Could you check a few things on this drawing? It's one solid part, dimensions in mm from its lowest x, y, z. Give positions to 0.01 mm unless a question says otherwise; leave off trailing zeros. Order: outer loops, then holes, each group sorted by start corner. A loop starts at its lowest first (then second) coordinate and runs counter-clockwise, first axis right, second up.
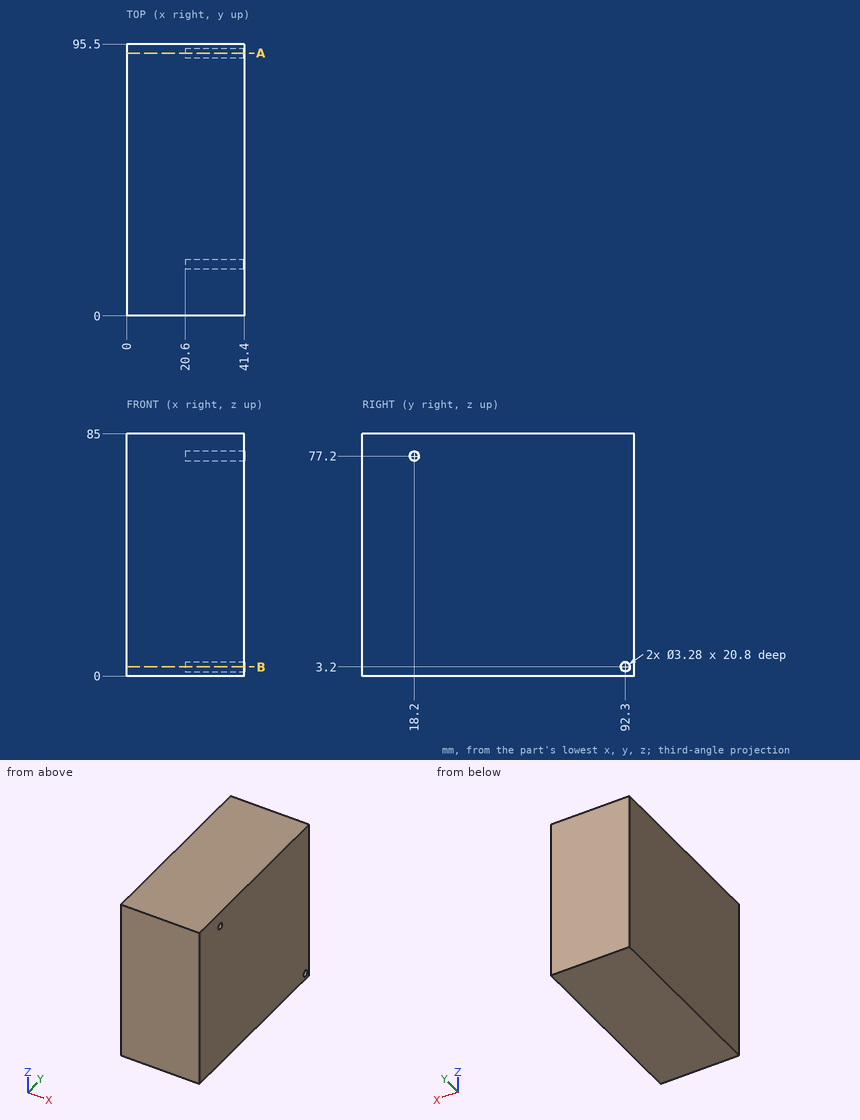
Item 1: Please list where these lines run through material, in increasing order: line 1 along Z through (x, y) = (32, 18); line 2 along Y through (x, z) = (30.5, 77.2); line 3 along Z through (x, y) = (34, 92).
Findings:
line 1: z = 0 to 75.57, 78.83 to 85
line 2: y = 0 to 16.56, 19.84 to 95.5
line 3: z = 0 to 1.59, 4.81 to 85
Item 2: Imagine slicing it at B-B on z = 3.2. List the corners of the cut face in (x, y) for me.
Findings:
outline: (0, 0) - (41.4, 0) - (41.4, 90.66) - (20.6, 90.66) - (20.6, 93.94) - (41.4, 93.94) - (41.4, 95.5) - (0, 95.5) - close
Item 3: Imagine slicing it at A-A on y = 92.3. List the corners of the cut face in (x, z) for me.
Findings:
outline: (0, 0) - (41.4, 0) - (41.4, 1.56) - (20.6, 1.56) - (20.6, 4.84) - (41.4, 4.84) - (41.4, 85) - (0, 85) - close
